Autodesk Inventor part; units mm, degrees
ref_plane "YZ Plane" through (0, 0, 0) normal (1, 0, 0) x (0, 1, 0)
ref_plane "XZ Plane" through (0, 0, 0) normal (0, 1, 0) x (-1, 0, 0)
ref_plane "XY Plane" through (0, 0, 0) normal (0, 0, 1) x (1, 0, 0)
sketch "Sketch1" plane through (0, 0, 0) normal (0, 0, 1) x (1, 0, 0)
  line L0 (-80, 40) -> (80, 40)
  line L1 (80, 40) -> (80, -40)
  line L2 (80, -40) -> (-80, -40)
  line L3 (-80, -40) -> (-80, 40)
  arc A0 (94, -60) -> (100, -54) centre (94, -54) ccw
  line L4 (94, -60) -> (-94, -60)
  arc A1 (-100, -54) -> (-94, -60) centre (-94, -54) ccw
  line L5 (-100, -54) -> (-100, 54)
  arc A2 (-94, 60) -> (-100, 54) centre (-94, 54) ccw
  line L6 (-94, 60) -> (94, 60)
  arc A3 (100, 54) -> (94, 60) centre (94, 54) ccw
  line L7 (100, 54) -> (100, -54)
  circle A4 centre (20, -30) radius 1.5
  circle A5 centre (-60, -30) radius 1.5
  circle A6 centre (20, 30) radius 1.5
  circle A7 centre (-60, 30) radius 1.5
  circle A8 centre (0, -31) radius 4
  circle A9 centre (50, 10) radius 21
  point P0 (0, 0)
  dimension "d0" = 20
  dimension "d1" = 20
  dimension "d2" = 20
  dimension "d3" = 20
  dimension "d19" = 160
  dimension "d20" = 80
extrude "Extrusion1" add sketch "Sketch1" along normal blind 1.5 contours L0 L1 L2 L3 | A8 | A9
sketch "Sketch2" plane through (0, 0, 1.5) normal (0, 0, 1) x (1, 0, 0)
  circle A0 centre (-70, 30) radius 5
  line L0 (80, 40) -> (-80, 40)
  line L1 (-80, 40) -> (-80, -40)
  circle A1 centre (-50, 30) radius 5
  circle A2 centre (-30, 30) radius 5
  circle A3 centre (-10, 30) radius 5
  circle A4 centre (10, 30) radius 5
  circle A5 centre (30, 30) radius 5
  circle A6 centre (50, 30) radius 5
  circle A7 centre (70, 30) radius 5
  circle A8 centre (-70, 10) radius 5
  circle A9 centre (-50, 10) radius 5
  circle A10 centre (-30, 10) radius 5
  circle A11 centre (-10, 10) radius 5
  circle A12 centre (10, 10) radius 5
  circle A13 centre (30, 10) radius 5
  circle A14 centre (50, 10) radius 5
  circle A15 centre (70, 10) radius 5
  circle A16 centre (-70, -10) radius 5
  circle A17 centre (-50, -10) radius 5
  circle A18 centre (-30, -10) radius 5
  circle A19 centre (-10, -10) radius 5
  circle A20 centre (10, -10) radius 5
  circle A21 centre (30, -10) radius 5
  circle A22 centre (50, -10) radius 5
  circle A23 centre (70, -10) radius 5
  circle A24 centre (-70, -30) radius 5
  circle A25 centre (-50, -30) radius 5
  circle A26 centre (-30, -30) radius 5
  circle A27 centre (-10, -30) radius 5
  circle A28 centre (10, -30) radius 5
  circle A29 centre (30, -30) radius 5
  circle A30 centre (50, -30) radius 5
  circle A31 centre (70, -30) radius 5
  point P0 (0, 0)
  dimension "d6" = 10
  dimension "d7" = 10
  dimension "d8" = 10
  dimension "d11" = 20
  dimension "d14" = 20
extrude "Extrusion2" cut sketch "Sketch2" against normal through all
fillet "Fillet1" radius 5 4 edges at (-80, -40, 0.75) (-80, 40, 0.75) (80, 40, 0.75) (80, -40, 0.75)
equation "\"d17\" = d14"
properties part number "sita"
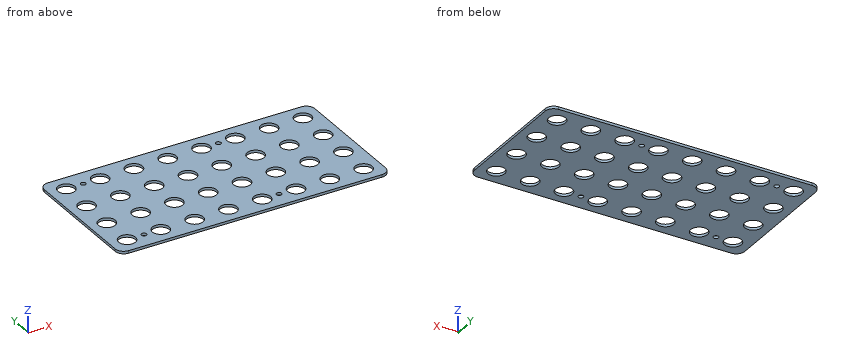
Geometry check sheet. Reference: the model listing, model coordinates, mm. Round coordinates to 2 decimals unless told otherwise and drop trailing zeros. Loops run counter-clockwise (first coordinate to the right, second up) from the corner with the lowest first, then second, coordinate; pieces in that order, holes last. Notation, with made-up numbers: M 30,88 L 73,88 A31 cw 73,120 Z; hole C 49,56.25 d1. An arc over 180 degrees is marked long. Return JSON: item names as keys, results as strings. Group by question number.
(1) Section check D-D, the plane x = -26.5. Enter the section's corners in (y, z), and give its area (3 significant figures).
(2) Go/stop test with flat-tipped pins: pin 1 (13 mm diameter, centred on x = -70, y = 10, fed in from +Z); pin 2 (9 mm diameter, centred on x = -70, y = -30, fed in from +Z). Record where each tip stops, or that it passes through.
(3) Scan lines: line 1 along Y through (x, z) = (-50, 0.85); line 2 along Y through (x, z) = (20, 1.25); line 3 along Y through (x, z) = (65.5, 0.45). Record each from-to range of solid material in increasing order. Write a range as [from, to].
(4) Section check A-A, the plane x = 30. Enter the section's corners in (y, z), and give its area (3 significant figures).
(5) Section check B-B, the plane y = -30. Give the number of separate pieces and of enclosed holes in the cut face, and give its area (3 significant figures).
Data:
{
 "1": {"outline": "M -40,0 L -33.57,0 L -33.57,1.5 L -40,1.5 Z; M -26.43,0 L -13.57,0 L -13.57,1.5 L -26.43,1.5 Z; M -6.43,0 L 6.43,0 L 6.43,1.5 L -6.43,1.5 Z; M 13.57,0 L 26.43,0 L 26.43,1.5 L 13.57,1.5 Z; M 33.57,0 L 40,0 L 40,1.5 L 33.57,1.5 Z", "area": "77.2 mm²"},
 "2": {"pin 1": "z = 1.5", "pin 2": "through"},
 "3": {"line 1": "[-40, -35], [-25, -15], [-5, 5], [15, 25], [35, 40]", "line 2": "[-40, -31.5], [-28.5, 28.5], [31.5, 40]", "line 3": "[-40, -32.18], [-27.82, -12.18], [-7.82, 7.82], [12.18, 27.82], [32.18, 40]"},
 "4": {"outline": "M -40,0 L -35,0 L -35,1.5 L -40,1.5 Z; M -25,0 L -15,0 L -15,1.5 L -25,1.5 Z; M -5,0 L 5,0 L 5,1.5 L -5,1.5 Z; M 15,0 L 25,0 L 25,1.5 L 15,1.5 Z; M 35,0 L 40,0 L 40,1.5 L 35,1.5 Z", "area": "60.0 mm²"},
 "5": {"separate pieces": "11", "enclosed holes": "0", "area": "111 mm²"}
}
